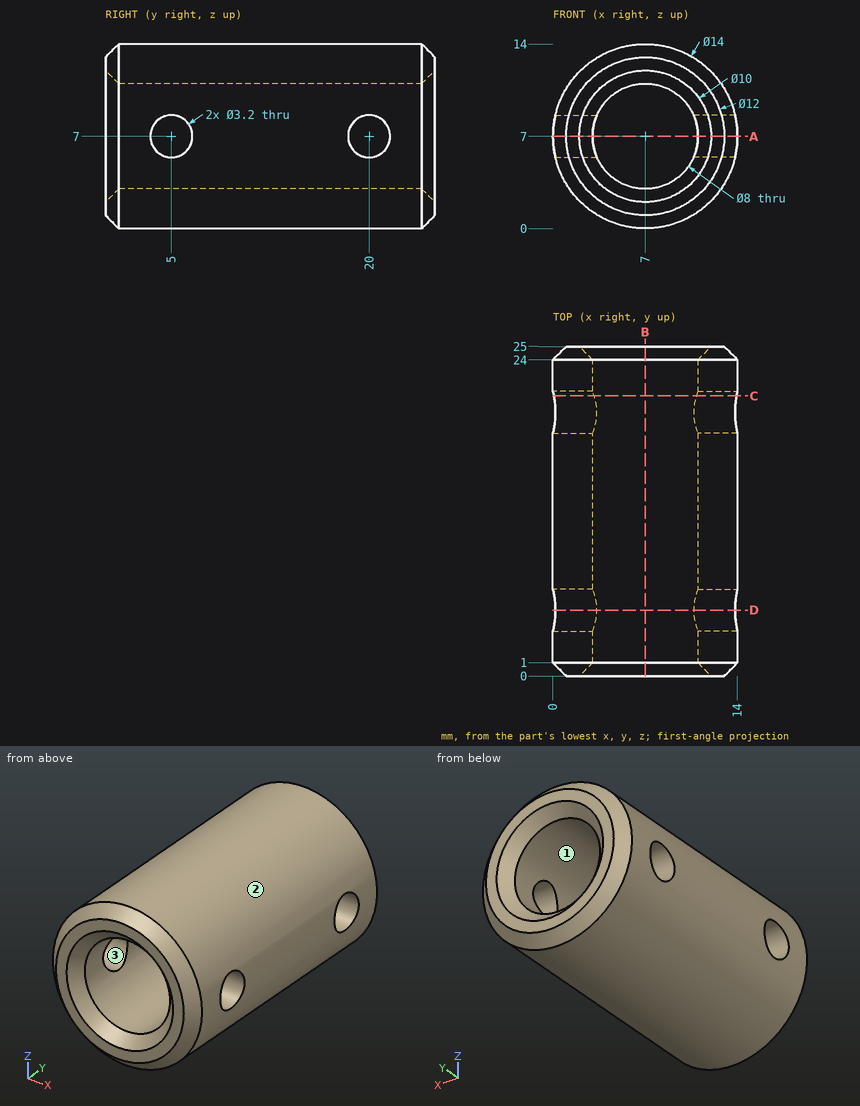
Study the drawing (mm; zero at the part's minimum x, y, z) and answer. Give positions to 0.01 mm unless a question says otherwise; leave off trailing zeros. Write each loop counter-clockwise with the first axis right and the second up, starting at its lowest first coordinate (ties: lowest second). Pieces come first, ordered by that corner, then holes. Notation, with made-up numbers: M -18,-39 L -9,-39 A15 ccw -9,-33 Z; hole C 39,-4 d7. An arc over 180 degrees is marked long. Put each result on its own line as item: value. Start each with the question number.
1. Each of these flat-tipped pins is pushed along its axis until it touches: pin 1 Ø5 at (y, z) = (19.5, 3) entering from -X; pin 2 Ø2.5 at (y, z) = (20, 7) entering from +X; pin 3 Ø6 at (x, y) = (9, 9) entering from +Z; pin 4 Ø1 at (x, y) = (8.5, 22) entering from -Z. Where does it stop, or does it pass through?
2. The part is cut by section B-B, the plane x = 7. Give the vertices of the cut face in (y, z), and give its area (3 significant figures).
3. The part is cut by section A-A, the plane z = 7. Give the number of separate pieces and of enclosed holes in the cut face, and give its area (3 significant figures).
4. Consider line 1 along Z through (x, y) = (11.85, 20); line 2 along X through (y, z) = (17.5, 7.25); line 3 along Z through (x, y) = (7.5, 23.5). Determine where each line is inside the solid, lowest interval first.
5. The part is cut by section C-C, the plane y = 21.25. Give the vertices of the cut face in (x, z), and give its area (3 significant figures).
6. For a pull along X with two mould halves and no side action, classify the marked faces 1, 2 and 3 as released by +X, released by -X, zero draft, split by the parting line, or undercut.
7. The part is cut by section D-D, the plane y = 5. Give the vertices of the cut face in (x, z), and give its area (3 significant figures).
Final values:
1. pin 1: stops at x = 0.16
1. pin 2: passes through
1. pin 3: stops at z = 14
1. pin 4: stops at z = 0.07
2. outline: M 0,1 L 1,0 L 24,0 L 25,1 L 25,2 L 24,3 L 1,3 L 0,2 Z; M 0,12 L 1,11 L 24,11 L 25,12 L 25,13 L 24,14 L 1,14 L 0,13 Z
2. area: 146 mm²
3. separate pieces: 6
3. enclosed holes: 0
3. area: 108 mm²
4. line 1: z = 1.95 to 5.4, 8.6 to 12.05
4. line 2: x = 0 to 3.01, 10.99 to 14
4. line 3: z = 0.02 to 3.03, 10.97 to 13.98
5. outline: M 0.07,6 A7 ccw 13.93,6 L 10.87,6 A4 cw 3.13,6 Z; M 0.07,8 L 3.13,8 A4 cw 10.87,8 L 13.93,8 A7 ccw Z
5. area: 91.6 mm²
6. face 1: undercut
6. face 2: split by the parting line
6. face 3: zero draft
7. outline: M 0.19,5.4 A7 ccw 13.81,5.4 L 10.67,5.4 A4 cw 3.33,5.4 Z; M 0.19,8.6 L 3.33,8.6 A4 cw 10.67,8.6 L 13.81,8.6 A7 ccw Z
7. area: 84.2 mm²
